Study the drawing (mm; zero at the part's minimum x, y, z) and answer. Give positions to 0.01 mm unless a question says otherwise; leave off trailing zeros. Write each loop counter-clockwise with the first axis right and the second up, starting at its lowest first coordinate (ties: lowest second). Pieces come first, ordered by that corner, then holes. Notation, with made-up numbers: M 49,37.5 L 59,37.5 A24 cw 59,72.5 Z; hole C -2,-7.5 d6. An arc over 180 degrees is marked long. Use a Markdown table: item, result. Add a question column.
Item 1: A cutting plane is placed at B-B on x = 6.35. Determine the outline of the cut face in (y, z), then the cut area to 3 significant figures.
Item 2: A cutting plane is placed at C-C on y = 3.25. Count the separate pieces of the cut face and the enclosed holes in it, then the cut area to 3 significant figures.
Item 3: Consider probe 1 along Z at (x, y) = (6.35, 3); probe 2 along X at (y, z) = (4.5, 31.75); probe 3 along X at (y, z) = (2.5, 21). Determine where each line is inside the solid, lowest interval first. Write a range as [from, to].
Item 4: Given P1, Ø2, axis at y = 3.5, z = 16, coming from the +X side; P2, Ø2, axis at x = 106, y = 3.5, coming from the -Z side, each flat-ended and moving along its own axis, determine where each tip first touches the part or whether it passes through.
Item 5: A cutting plane is placed at A-A on z = 31.75. Determine the outline of the cut face in (x, y), then the cut area to 3 significant figures.
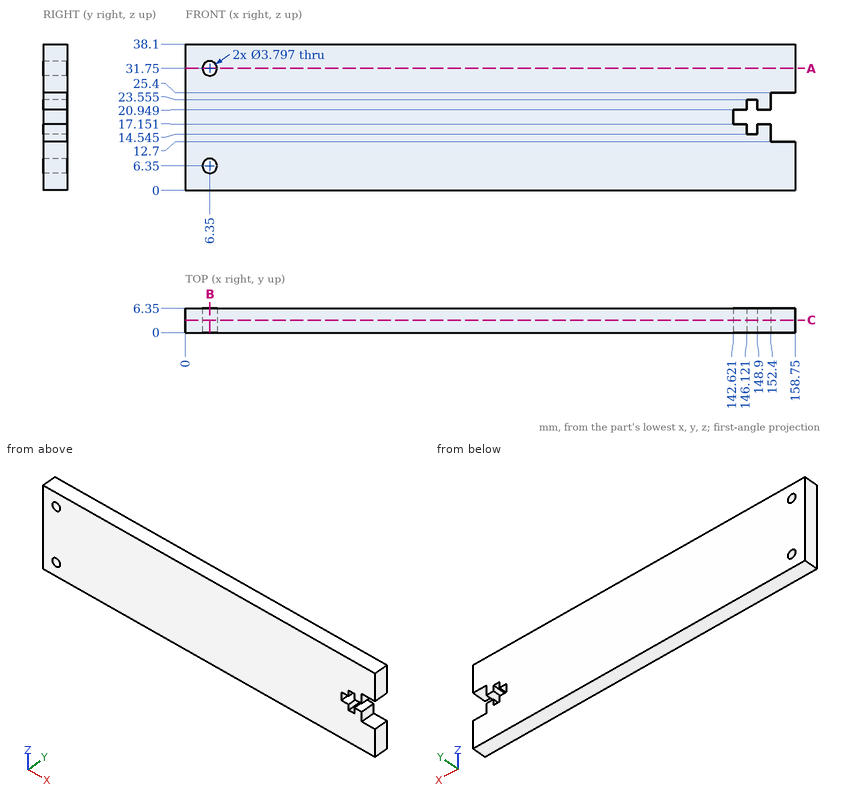
Filled in:
| question | item | result |
|---|---|---|
| 1 | outline | M 0,0 L 6.35,0 L 6.35,4.45 L 0,4.45 Z; M 0,8.25 L 6.35,8.25 L 6.35,29.85 L 0,29.85 Z; M 0,33.65 L 6.35,33.65 L 6.35,38.1 L 0,38.1 Z |
| 1 | area | 194 mm² |
| 2 | separate pieces | 1 |
| 2 | enclosed holes | 2 |
| 2 | area | 5,890 mm² |
| 3 | probe 1 | [0, 4.45], [8.25, 29.85], [33.65, 38.1] |
| 3 | probe 2 | [0, 4.45], [8.25, 158.75] |
| 3 | probe 3 | [0, 146.12], [148.9, 152.4] |
| 4 | P1 | x = 152.4 |
| 4 | P2 | z = 0 |
| 5 | outline | M 0,0 L 4.45,0 L 4.45,6.35 L 0,6.35 Z; M 8.25,0 L 158.75,0 L 158.75,6.35 L 8.25,6.35 Z |
| 5 | area | 984 mm² |
